CAD build for the part. Positions are in the model's coordinates, mm. A direction names the side the tool comes from. Round coordinates to 2 decimals unless told otherwise and drop trailing zeros. Write each loop counter-clockwise with the first axis right and the second up, starting at its lowest first coordinate (ties: lowest second). Pieces come first, ordered by that corner, then holes. Notation, with made-up numbers: M 85,73.25 L 98,73.25 A17 cw 98,100.25 Z; hole C -18.75,-19.75 d10. An arc over 180 degrees is marked long. Write each question's results on one line, items separated by ' | '. Start each with the question number.
Autodesk Inventor part; units mm, degrees
ref_plane "YZ Plane" through (0, 0, 0) normal (1, 0, 0) x (0, 1, 0)
ref_plane "XZ Plane" through (0, 0, 0) normal (0, 1, 0) x (-1, 0, 0)
ref_plane "XY Plane" through (0, 0, 0) normal (0, 0, 1) x (1, 0, 0)
sketch "Sketch1" plane through (0, 0, 0) normal (0, 0, 1) x (1, 0, 0)
  line L0 (15, 0) -> (12.5, 0)
  line L1 (12.5, 0) -> (12.5, 4)
  line L2 (2.5, 4) -> (2.5, 0)
  line L3 (2.5, 0) -> (0, 0)
  line L4 (12.5, 4) -> (9.0875, 4)
  line L5 (9.0875, 4) -> (9.0875, 97)
  line L6 (9.0875, 97) -> (5.9125, 97)
  line L7 (5.9125, 97) -> (5.9125, 4)
  line L8 (5.9125, 4) -> (2.5, 4)
  line L9 (0, 194) -> (2.5, 194)
  line L10 (2.5, 194) -> (2.5, 190)
  line L11 (2.5, 190) -> (12.5, 190)
  line L12 (12.5, 190) -> (12.5, 194)
  line L13 (12.5, 194) -> (15, 194)
  line L14 (0, 194) -> (0, 188)
  line L15 (0, 188) -> (3.25, 184.75)
  line L16 (3.25, 184.75) -> (3.25, 9.25)
  line L17 (0, 0) -> (0, 6)
  line L18 (0, 6) -> (3.25, 9.25)
  line L19 (15, 0) -> (15, 6)
  line L20 (15, 6) -> (11.75, 9.25)
  line L21 (11.75, 9.25) -> (11.75, 184.75)
  line L22 (11.75, 184.75) -> (15, 188)
  line L23 (15, 188) -> (15, 194)
  dimension "d1" = 10
  dimension "d2" = 3.175
  dimension "d4" = 194
  dimension "d7" = 97
  dimension "d10" = 6
  dimension "d13" = 15
  dimension "d14" = 45
  dimension "d15" = 4
  dimension "d16" = 8.5
extrude "Extrusion1" add sketch "Sketch1" along normal blind 3.175
equation "\"d2\" = THICKA"
equation "\"d7\" = 0.5 * d4"
equation "\"d8\" = THICKA"
equation "\"THICKA\" = 3.175"
equation "\"THICKB\" = 6.731"
equation "\"THICKC\" = 12.7"
properties part number "Effector_Arm"
1) Pull direction Y, two halves, no side cores. Call faces 4 (the face through (2, 8, 2)), 5 (the face through (11, 4, 2)), 6 (the face through (0, 3, 2)): pulls with the +Y half, pulls with the -Y half, needs draft (parallel to the pull), parting line crosses it, or undercut.
2) Drop flat-ended pins along their axis: pin 1 Ø8 at (x, y) = (2.5, 126) entering from +Z (3 decimals); pin 2 Ø1.5 at (y, z) = (47, 0.5) entering from -X; pin 3 Ø1 at (x, z) = (8.5, 2) entering from +Y; pin 4 Ø1.6 at (x, z) = (3.5, 1) entering from -Y. Give the stop position or say it passes through.
3) Saw through at C-C, the plane y = 146. Write the cut outline in (x, z) (3 decimals), plus the area to 3 significant figures.
4) Saw through at B-B, the plane z = 2.5. Write the cut outline in (x, y).
5) Wall check: line 1 along X through (y, z) = (42, 0.4); line 2 along Y through (x, z) = (6.5, 0.4); line 3 along X through (y, z) = (9, 3). Give the ranges that are in metal, low to high. Write a range as from..to.
6) 3-axis set-ups, long thin cutter, end or side, ignore diameter. For faces 1 (the face through (13, 8, 2)), 2 (the face through (12.5, 2, 2)), 3 (the face through (3.25, 98, 2)): which of +Z, -Z, +X, -X, +Y, -Y reach the whole face in a straight line?
Filled sheet:
1) face 4: undercut | face 5: pulls with the -Y half | face 6: needs draft
2) pin 1: stops at z = 3.175 | pin 2: stops at x = 3.25 | pin 3: stops at y = 190 | pin 4: stops at y = 4
3) outline: M 3.25,0 L 11.75,0 L 11.75,3.175 L 3.25,3.175 Z | area: 27.0 mm^2
4) outline: M 0,0 L 2.5,0 L 2.5,4 L 5.91,4 L 5.91,97 L 9.09,97 L 9.09,4 L 12.5,4 L 12.5,0 L 15,0 L 15,6 L 11.75,9.25 L 11.75,184.75 L 15,188 L 15,194 L 12.5,194 L 12.5,190 L 2.5,190 L 2.5,194 L 0,194 L 0,188 L 3.25,184.75 L 3.25,9.25 L 0,6 Z
5) line 1: x = 3.25..5.91, 9.09..11.75 | line 2: y = 97..190 | line 3: x = 3..5.91, 9.09..12
6) face 1: +Z, -Z, +X | face 2: +Z, -Z, -Y | face 3: +Z, -Z, -X
